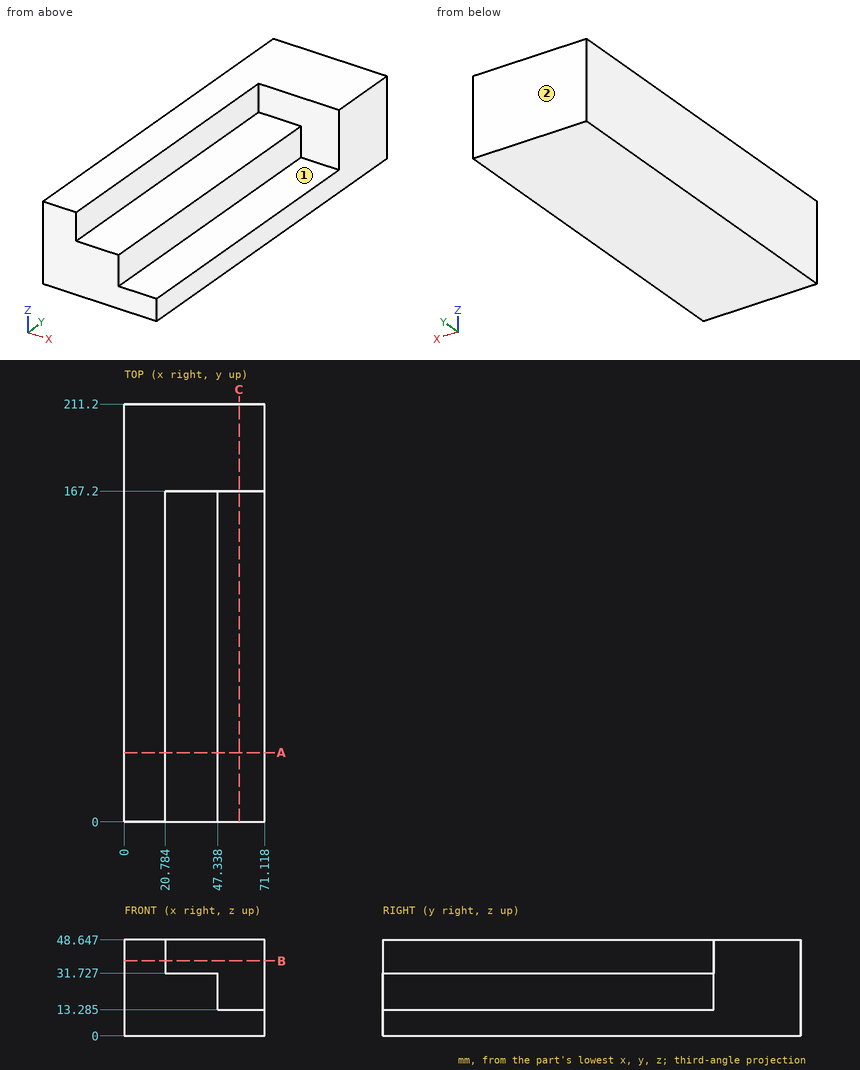
Print and shaded views of the part. All mm, measured from the part's lowest x, y and z. A direction names the side the tool comes from. Coordinates: 2 decimals unless noted, no trailing zeros. Order: outer loops, then holes, each group sorted by start corner. A loop starts at its lowest first (then second) coordinate and runs counter-clockwise, first axis right, second up. Notation, with made-up numbers: M -23,75.5 L 10,75.5 A13 ccw 10,94.5 Z; hole C 12,-35.75 d8. An arc over 180 degrees is marked long. One line per question, with ' | ' between items. Start each with the question number.
Q1. Saw through at C-C (x = 58). List the corners of the cut face in (y, z) (1 decimal), then the cut area to 3 significant figures.
Q2. Probe L1, parallel to Z at x = 41, y = 103; L2, parallel to Y at x = 40.5, z = 46; L3, parallel to X at y = 94, z = 19. List the from-to ranges inside material, lowest first. Write a range as from..to.
Q3. Saw through at B-B (z = 38). List the corners of the cut face in (x, y).
Q4. Saw through at A-A (y = 35). List the corners of the cut face in (x, z) (1 decimal), then the cut area to 3 significant figures.
Q5. Flat gauge pins, fed straight in: pin 1 Ø8.5 at (y, z) = (123, 43) entering from +X; pin 2 Ø21 at (x, y) = (33, 117.5) entering from +Z; pin 3 Ø12 at (x, y) = (56, 102) entering from +Z (1 decimal). Where does each tip first touch, or does it go through?
Q6. 3-axis set-ups, long thin cutter, end or side, ignore diameter. For the marked faces 1 and 2: which of +Z, -Z, +X, -X, +Y, -Y reach the whole face in a straight line?
Check values:
1) outline: M 0,0 L 211.2,0 L 211.2,48.6 L 167.2,48.6 L 167.2,13.3 L 0,13.3 Z | area: 4,360 mm2
2) L1: z = 0..31.73 | L2: y = 167.2..211.2 | L3: x = 0..47.34
3) outline: M 0,0 L 20.78,0 L 20.78,167.2 L 71.12,167.2 L 71.12,211.2 L 0,211.2 Z
4) outline: M 0,0 L 71.1,0 L 71.1,13.3 L 47.3,13.3 L 47.3,31.7 L 20.8,31.7 L 20.8,48.6 L 0,48.6 Z | area: 2,170 mm2
5) pin 1: stops at x = 20.78 | pin 2: stops at z = 31.73 | pin 3: stops at z = 13.3
6) face 1: +Z, +X, -Y | face 2: +Z, -Z, +X, -X, +Y
